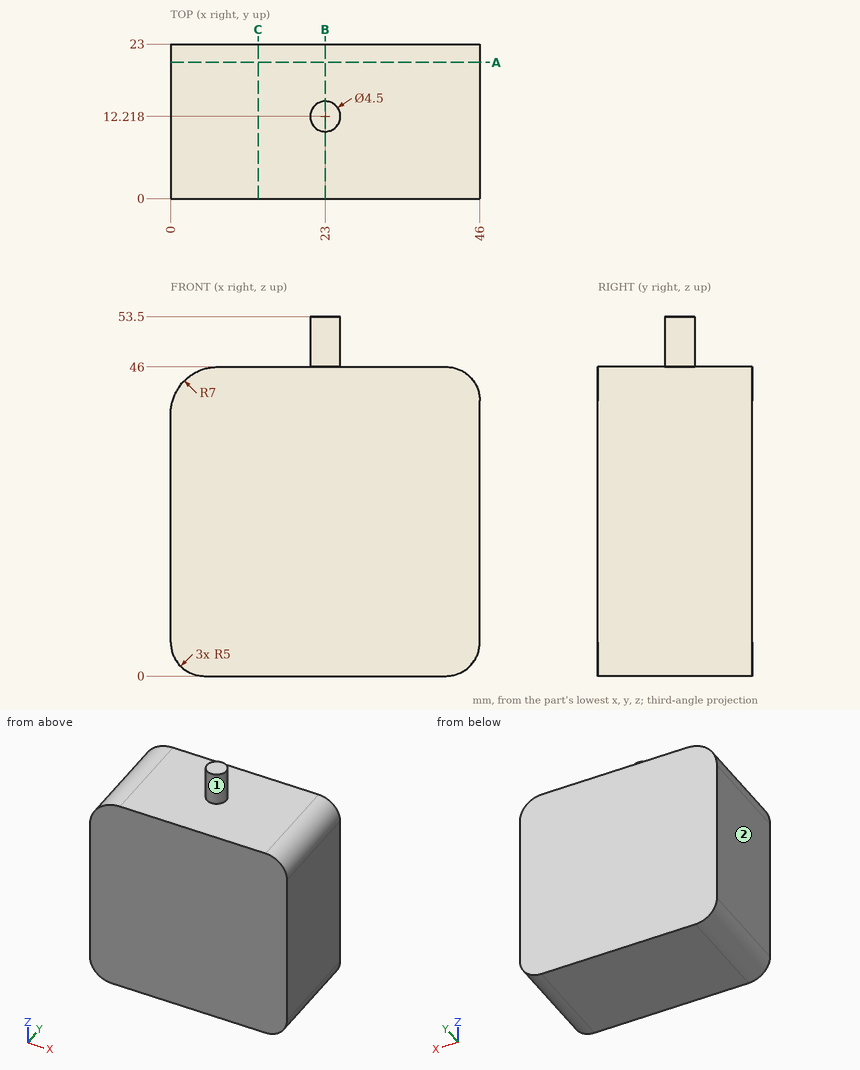
Answer from the drawing. Dimensions are ordinates in mm from the lowest x, y and z of the part. A direction names the side the tool comes from. Give positions to 0.01 mm unless a question says otherwise; leave off trailing zeros. Loops run counter-clockwise (first coordinate to the right, second up) from the corner with the lowest first, then second, coordinate; pieces in that order, holes last.
Item 1: The part is cut by section A-A (y = 20.25). Write down the section's boundary in (x, z), and give its area (3 significant figures).
Item 2: The part is cut by section C-C (x = 13). Write down the section's boundary in (y, z), and give its area (3 significant figures).
Item 3: The part is cut by section B-B (x = 23). Write down the section's boundary in (y, z), and give its area (3 significant figures).
Item 4: For the marked faces 1 and 2, determine the directions among +Z, -Z, +X, -X, +Y, -Y from which every point of the face is accessible in a straight line to the end or side of a thin tool.
Item 5: This flat-tipped pin is pushed along its axis until it touches: pin 1 Ø6 at (x, y) = (16.5, 14) entering from +Z. Where does it stop, or does it pass through?
Item 6: Find the intervals of material crossed by line 1 along Z through (x, y) = (7, 7.25); line 2 along X through (y, z) = (11.5, 40.5); line 3 along Z through (x, y) = (4, 8.5), in increasing order.
Taken from the geometry:
1. outline: (0, 5) arc R5 ccw to (5, 0) - (41, 0) arc R5 ccw to (46, 5) - (46, 41) arc R5 ccw to (41, 46) - (7, 46) arc R7 ccw to (0, 39) - close
1. area: 2,090 mm2
2. outline: (0, 0) - (23, 0) - (23, 46) - (0, 46) - close
2. area: 1,060 mm2
3. outline: (0, 0) - (23, 0) - (23, 46) - (14.47, 46) - (14.47, 53.5) - (9.97, 53.5) - (9.97, 46) - (0, 46) - close
3. area: 1,090 mm2
4. face 1: +Z
4. face 2: +Z, -Z, -X, +Y, -Y
5. pin 1: stops at z = 46
6. line 1: z = 0 to 46
6. line 2: x = 0.16 to 46
6. line 3: z = 0.1 to 45.32
